from build123d import *

# Parameters (mm, degrees)
BASPROSKE_W        = 11.811
BASPROSKE_H        = 28.575
TOOTHCUT_DEPTH     = 43.101792967
TEETHCUTS_COUNT    = 16
TEETHCUTS_ANGLE    = 337.5
BORSKE_R           = 0.396875
BORE_DEPTH         = 50.8000508
CUT_EXTRUDE1_DEPTH = 42.540449503


with BuildPart() as part:
    # BasProSke → Base-Revolve (revolve)
    with BuildSketch(Plane(origin=(0, 0, 0), x_dir=(1, 0, 0), z_dir=(0, 1, 0)), mode=Mode.PRIVATE) as base_revolve_sk:
        with Locations((5.9055, 14.2875)):
            Rectangle(BASPROSKE_W, BASPROSKE_H)
    revolve(base_revolve_sk.sketch.rotate(Axis((-10, 0, 0), (1, 0, 0)), 180), axis=Axis((-10, 0, 0), (1, 0, 0)))

    # TooCutSke → ToothCut (cut, through all)
    with BuildSketch(Plane(origin=(0, 0, 0), x_dir=(0, 0, -1), z_dir=(1, 0, 0))):
        with BuildLine():
            ThreePointArc((1.653773222, 21.366073035), (0, 21.42998), (-1.653773222, 21.366073035))
            ThreePointArc((-1.653773222, 21.366073035), (-2.605634946, 25.083646688), (-4.868483936, 28.182986789))
            ThreePointArc((-4.868483936, 28.182986789), (0, 28.6004), (4.868483936, 28.182986789))
            ThreePointArc((4.868483936, 28.182986789), (2.605634946, 25.083646688), (1.653773222, 21.366073035))
        make_face()
    toothcut = extrude(amount=TOOTHCUT_DEPTH, mode=Mode.SUBTRACT)

    # TeethCuts: ToothCut ×16 about axis
    teethcuts_axis = Axis((-10, 0, 0), (1, 0, 0))
    for i in range(1, TEETHCUTS_COUNT):
        add(toothcut.rotate(teethcuts_axis, i * TEETHCUTS_ANGLE / (TEETHCUTS_COUNT - 1)), mode=Mode.SUBTRACT)

    # BorSke → Bore (cut, symmetric)
    with BuildSketch(Plane(origin=(0, 0, 0), x_dir=(0, 0, -1), z_dir=(1, 0, 0))):
        with Locations(Location((0, 0, 0), (0, 0, 180))):
            Circle(BORSKE_R)
    extrude(amount=BORE_DEPTH, both=True, mode=Mode.SUBTRACT)

    # Sketch1 → Cut-Extrude1 (cut, through all)
    with BuildSketch(Plane(origin=(11.811, 0, 0), x_dir=(0, 0, -1), z_dir=(1, 0, 0))):
        with BuildLine():
            Line((-1.658312395, 2.5), (1.658312395, 2.5))
            ThreePointArc((1.658312395, 2.5), (0, -3), (-1.658312395, 2.5))
        make_face()
    extrude(amount=-CUT_EXTRUDE1_DEPTH, mode=Mode.SUBTRACT)


solid = part.part
Part model, mm, in its own coordinate system. A direction names the side the tool comes from. Round coordinates to 2 decimals unless told otherwise and drop trailing zeros. Loops run counter-clockwise (first coordinate to the right, second up) from the corner with the lowest first, then second, coordinate; pieces in that order, holes last. Notation, with made-up numbers: (51, -27.75) - (108, -27.75) arc R18 cw to (108, 5.25) - close; hole circle Ø3 at (-10, 68). An arc over 180 degrees is marked (long way). Answer as a JSON object with one key per item and string values.
Item 1: Band-saw the part on A-A on z = 0. List the corners of the cut face in (x, y).
Output:
{"outline": "(0, -21.43) - (11.81, -21.43) - (11.81, -3) - (0, -3) - close; (0, 2.5) - (11.81, 2.5) - (11.81, 21.43) - (0, 21.43) - close"}
Item 2: Pull direction Y, two halves, no side cores. Call faces 1 (the face through (5.82, 19.51, -15.87)), 2 (the face through (5.823, 25.02, 2.576)), 3 (the face through (5.82, -12.03, -22.2)), 4 (the face through (5.823, -25.02, -2.576)): pulls with the +Y half, pulls with the -Y half, needs draft (parallel to the pull), parting line crosses it, or undercut.
Output:
{"face 1": "undercut", "face 2": "pulls with the +Y half", "face 3": "undercut", "face 4": "pulls with the -Y half"}
Item 3: Tool access for faces 5 (the face through (5.823, -15.17, -15.137)), 6 (the face through (5.823, -2.576, 25.02)), 7 (the face through (5.823, -2.622, -25.118)): list every direction of +Z, -Z, +X, -X, +Y, -Y with a clear straight run to the whole face (end or side of a thin tool).
Output:
{"face 5": "+X, -X", "face 6": "+Z, +X, -X", "face 7": "-Z, +X, -X"}
Item 4: Wall check: L1, parallel to Y at x = 7.25, z = -22; L2, parallel to Z at x = 5.25, y = 0; L3, parallel to Z at x = 7.25, y = -23. Give the ranges that are in metal, low to high.
Output:
{"L1": "-16.44 to -11.82, -7.06 to -1.71, 1.71 to 7.06, 11.82 to 16.44", "L2": "-21.43 to -3, 3 to 21.43", "L3": "-16.49 to -13.04, -7.18 to -1.89, 1.89 to 7.18, 13.04 to 16.49"}
Item 5: Pin check, flat tips, straight feed: pin 1 (2 mm diameter, centred on y = 19, z = -9, fed in from -X); pin 2 (1 mm diameter, centred on x = 3, z = 8, fed in from +Y); pin 3 (6 mm diameter, centred on x = 6.5, z = 2, fed in from +Y); pin 4 (2 mm diameter, centred on y = 22, z = 8.5, fed in from -X). Stop position of each tip, or through.
Output:
{"pin 1": "x = 0", "pin 2": "y = 20.07", "pin 3": "y = 28.16", "pin 4": "through"}
Item 6: Band-saw the part on B-B on y = 0. List the corners of the cut face in (x, z), plus the area to 3 significant figures.
Output:
{"outline": "(0, -21.43) - (11.81, -21.43) - (11.81, -3) - (0, -3) - close; (0, 3) - (11.81, 3) - (11.81, 21.43) - (0, 21.43) - close", "area": "435 mm2"}
Item 7: Band-saw the part on D-D on z = 17.5. List the corners of the cut face in (x, y), plus the area to 3 significant figures.
Output:
{"outline": "(0, -14.87) - (11.81, -14.87) - (11.81, 14.87) - (0, 14.87) - close", "area": "351 mm2"}
Item 8: Band-saw the part on C-C on z = -22.5. List the corners of the cut face in (x, y).
Output:
{"outline": "(0, -16.48) - (11.81, -16.48) - (11.81, -12.38) - (0, -12.38) - close; (0, -7.13) - (11.81, -7.13) - (11.81, -1.79) - (0, -1.79) - close; (0, 1.79) - (11.81, 1.79) - (11.81, 7.13) - (0, 7.13) - close; (0, 12.38) - (11.81, 12.38) - (11.81, 16.48) - (0, 16.48) - close"}
